```python
from build123d import *

# Parameters (mm, degrees)
F2_R = 5.08
F3_R = 5.08


with BuildPart() as f1:
    # F0 (on Front) → F1 (revolve)
    with BuildSketch(Plane.XZ):
        Polygon((0, -50.344978), (0, 28.951926), (-12.835828, 28.951926), (-15.688237, 21.82091), (-9.983422, 21.82091), (-12.835828, 17.257059), (-19.966844, 17.257059), (-24.508418, -3.180023), (-27.346618, -16.265895), (-27.346618, -50.344978), align=None)
    revolve(axis=Axis((0, 0, -10.696526), (0, 0, 1)))

    # F2
    f2_edges = [f1.edges().sort_by_distance(p)[0] for p in [
        (19.966844, 0, 17.257059),
        (24.508418, 0, -3.180023),
        (-22.237631, 0, 7.038518),
    ]]
    fillet(f2_edges, radius=F2_R)

    # F3
    f3_edges = [f1.edges().sort_by_distance(p)[0] for p in [
        (27.346618, 0, -16.265895),
    ]]
    fillet(f3_edges, radius=F3_R)


solid = f1.part
```
Source: CAD feature listing. Evaluate the final solid. Frame: model axes, mm. A direction names the side the tool comes from. Give positions to 0.01 mm unless a question says otherwise; leave off trailing zeros. Loops run counter-clockwise (first coordinate to the right, second up) from the corner with the lowest first, then second, coordinate; pieces in that order, holes last. Notation, with made-up numbers: (36.25, 38.5) - (44.25, 38.5) arc R21 cw to (44.25, 77.5) - close; hole circle Ø5 at (56.25, -1). An arc over 180 degrees is marked (long way). Use CSV: the item, a comma, the result in double quotes.
1) Set-up query: faces 1 (the flat face through (-11, -7, 17.257)), 2 (the conical face through (4.658, 20.975, 10.421)). Return all of +Z, -Z, +X, -X, +Y, -Y with unobstructed straight access to the full face (end or side cutting, diameter ignored); none if empty.
Worked out:
face 1,"none"
face 2,"+Z"
2) Pin query (flat end, axial travel): P1, Ø3, axis at y = 4.5, z = 15, coming from the +X side; P2, Ø3, axis at x = -14, y = 14, coming from the +Z side; P3, Ø6, axis at x = 11.5, z = -11, coming from the +Y side. Return the tip coordinate at first contact, or that it passes through.
Worked out:
P1,"stops at x = 20.4"
P2,"stops at z = 16.65"
P3,"stops at y = 24.99"
3) Cut plane A-A (z = 7). Output: boundary loops of the cut face in (x, y).
Worked out:
outline,"circle Ø44.49 at (0, 0)"
4) Line query: line 1 (Z direction, x = -7.5, y = 7); line 2 (Z direction, x = -9.5, y = -8); line 3 (X direction, y = 18.5, z = -37.5). Output: solid intervals per line, ascending.
Worked out:
line 1,"z = -50.34 to 21.38, 21.82 to 28.95"
line 2,"z = -50.34 to 17.92, 21.82 to 28.95"
line 3,"x = -20.14 to 20.14"
